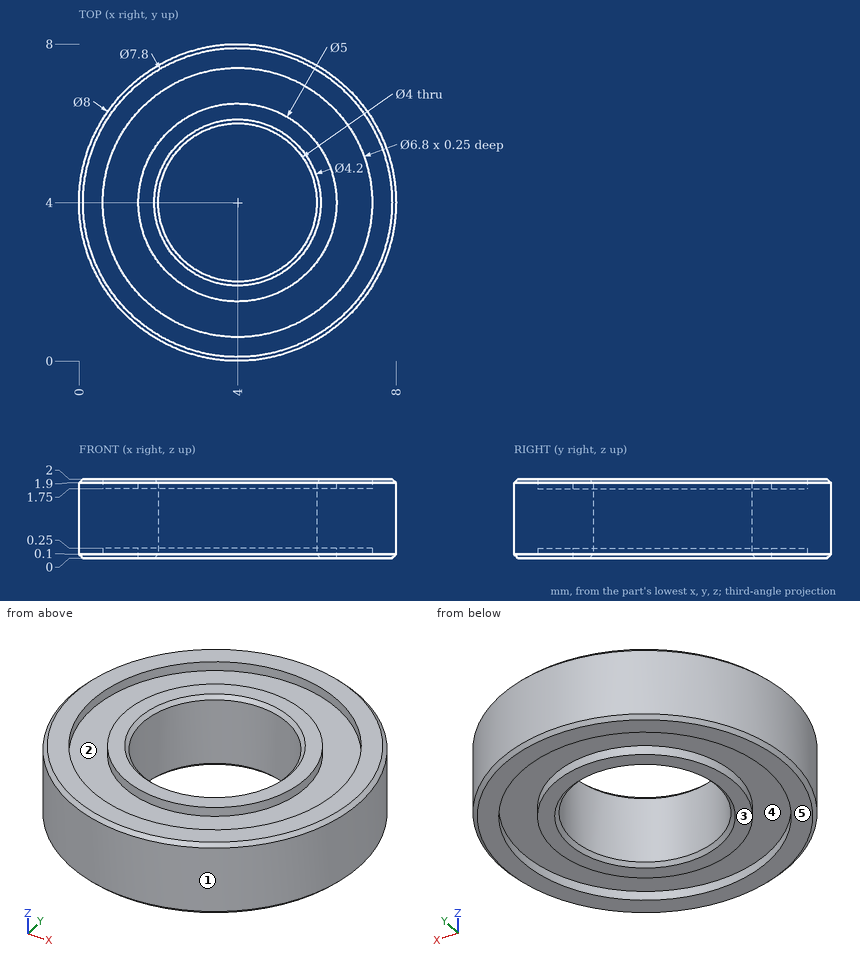
Drawing for the job (mm, zero at the part's lowest x, y, z). A direction names the side the tool comes from. Round coordinates to 2 decimals unless told otherwise and drop trailing zeros. Return JSON: item names as keys, results as strings. Group by question number.
Q1. Tool access for the marked faces 4 and 5: list every direction of +Z, -Z, +X, -X, +Y, -Y with a clear straight run to the whole face (end or side of a thin tool).
Q2. Two-plate mould, pull along X, no slides. Class the marked faces 1, 2 and 3: +X half, -X half, draft (parallel to the pull), parting line (faces both ways), or undercut.
Q3. Drill centre lines: line 1 along Y through (x, z) = (4, 0.6); line 2 along X through (y, z) = (3, 1.85). Where is each one in solid material? Low to high. Write a range as [from, to].
Solutions:
{
 "1": {"face 4": "-Z", "face 5": "-Z, +X, -X, +Y, -Y"},
 "2": {"face 1": "parting line", "face 2": "undercut", "face 3": "draft"},
 "3": {"line 1": "y = [0, 2], [6, 8]", "line 2": "x = [0.13, 0.75], [1.71, 2.27], [5.73, 6.29], [7.25, 7.87]"}
}
